```python
from build123d import *

# Parameters (mm, degrees)
BOSS_EXTRUDE1_DEPTH     = 35
CUT_EXTRUDE1_DEPTH      = 47.8508271
CUT_EXTRUDE1_DEPTH_BACK = 47.8508271
SKETCH2_R               = 12.8
SKETCH3_R               = 2
CUT_EXTRUDE2_DEPTH      = 7.5
SKETCH4_R               = 3.75
CUT_EXTRUDE3_DEPTH      = 16.5
SKETCH5_R               = 1.8
CUT_EXTRUDE4_DEPTH      = 22
SKETCH6_R               = 4
CUT_EXTRUDE5_DEPTH      = 2
SKETCH7_W               = 32
SKETCH7_H               = 6
CUT_EXTRUDE6_DEPTH      = 2
CUT_EXTRUDE7_DEPTH      = 47.850827224
CUT_EXTRUDE7_DEPTH_BACK = 47.850827224
SKETCH8_R               = 1.8
SKETCH9_R               = 3.75
CUT_EXTRUDE8_DEPTH      = 5
CUT_EXTRUDE9_DEPTH      = 8


with BuildPart() as part:
    # Sketch1 → Boss-Extrude1 (new, symmetric)
    with BuildSketch(Plane(origin=(0, 0, 0), x_dir=(0, 0, -1), z_dir=(1, 0, 0))):
        with BuildLine():
            Line((-19, 0.6), (19, 0.6))
            ThreePointArc((19, 0.6), (21.828427125, 1.771572875), (23, 4.6))
            Line((23, 4.6), (23, 17))
            ThreePointArc((23, 17), (21.828427125, 19.828427125), (19, 21))
            Line((19, 21), (-19, 21))
            ThreePointArc((-19, 21), (-21.828427125, 19.828427125), (-23, 17))
            Line((-23, 17), (-23, 4.6))
            ThreePointArc((-23, 4.6), (-21.828427125, 1.771572875), (-19, 0.6))
        make_face()
    extrude(amount=BOSS_EXTRUDE1_DEPTH, both=True)

    # Sketch2 → Cut-Extrude1 (cut, two sides: drawn at the far end of the back side and taken through both)
    with BuildSketch(Plane(origin=(0, 0, 0), x_dir=(0, 0, -1), z_dir=(1, 0, 0)).offset(-CUT_EXTRUDE1_DEPTH_BACK)):
        Circle(SKETCH2_R)
    extrude(amount=CUT_EXTRUDE1_DEPTH + CUT_EXTRUDE1_DEPTH_BACK, mode=Mode.SUBTRACT)

    # Sketch3 → Cut-Extrude2 (cut)
    with BuildSketch(Plane(origin=(0, 0.6, 0), x_dir=(1, 0, 0), z_dir=(0, 1, 0))):
        with Locations(Location((28, -17.5, 0), (0, 0, 228.590377891))):
            Circle(SKETCH3_R)
        with Locations(Location((28, 17.5, 0), (0, 0, 48.590377891))):
            Circle(SKETCH3_R)
        with Locations(Location((-28, -17.5, 0), (0, 0, 228.590377891))):
            Circle(SKETCH3_R)
        with Locations(Location((-28, 17.5, 0), (0, 0, 48.590377891))):
            Circle(SKETCH3_R)
    extrude(amount=CUT_EXTRUDE2_DEPTH, mode=Mode.SUBTRACT)

    # Sketch4 → Cut-Extrude3 (cut)
    with BuildSketch(Plane(origin=(0, 0, 0), x_dir=(1, 0, 0), z_dir=(0, 1, 0))):
        with Locations(Location((8.84, -8.84, 0), (0, 0, 90))):
            Circle(SKETCH4_R)
        with Locations(Location((8.84, 8.84, 0), (0, 0, 90))):
            Circle(SKETCH4_R)
        with Locations(Location((-8.84, -8.84, 0), (0, 0, 90))):
            Circle(SKETCH4_R)
        with Locations(Location((-8.84, 8.84, 0), (0, 0, 90))):
            Circle(SKETCH4_R)
    extrude(amount=CUT_EXTRUDE3_DEPTH, mode=Mode.SUBTRACT)

    # Sketch5 → Cut-Extrude4 (cut)
    with BuildSketch(Plane(origin=(0, 0, 0), x_dir=(1, 0, 0), z_dir=(0, 1, 0))):
        with Locations(Location((8.84, -8.84, 0), (0, 0, 90))):
            Circle(SKETCH5_R)
        with Locations(Location((8.84, 8.84, 0), (0, 0, 90))):
            Circle(SKETCH5_R)
        with Locations(Location((-8.84, -8.84, 0), (0, 0, 90))):
            Circle(SKETCH5_R)
        with Locations(Location((-8.84, 8.84, 0), (0, 0, 90))):
            Circle(SKETCH5_R)
    extrude(amount=CUT_EXTRUDE4_DEPTH, mode=Mode.SUBTRACT)

    # Sketch6 → Cut-Extrude5 (cut)
    with BuildSketch(Plane(origin=(0, 21, 0), x_dir=(1, 0, 0), z_dir=(0, 1, 0))):
        with Locations(Location((0, 0, 0), (0, 0, 270))):
            Circle(SKETCH6_R)
    extrude(amount=-CUT_EXTRUDE5_DEPTH, mode=Mode.SUBTRACT)

    # Sketch7 → Cut-Extrude6 (cut)
    with BuildSketch(Plane(origin=(0, 21, 0), x_dir=(1, 0, 0), z_dir=(0, 1, 0))):
        with Locations((19, 0)):
            Rectangle(SKETCH7_W, SKETCH7_H)
    extrude(amount=-CUT_EXTRUDE6_DEPTH, mode=Mode.SUBTRACT)

    # Sketch8 → Cut-Extrude7 (cut, two sides: drawn at the far end of the back side and taken through both)
    with BuildSketch(Plane.XY.offset(-CUT_EXTRUDE7_DEPTH_BACK)):
        with Locations((18, 0)):
            Circle(SKETCH8_R)
        with Locations((-18, 0)):
            Circle(SKETCH8_R)
    extrude(amount=CUT_EXTRUDE7_DEPTH + CUT_EXTRUDE7_DEPTH_BACK, mode=Mode.SUBTRACT)

    # Sketch9 → Cut-Extrude8 (cut)
    with BuildSketch(Plane.XY.offset(23)):
        with Locations((18, 0)):
            Circle(SKETCH9_R)
        with Locations((-18, 0)):
            Circle(SKETCH9_R)
    extrude(amount=-CUT_EXTRUDE8_DEPTH, mode=Mode.SUBTRACT)

    # Sketch10 → Cut-Extrude9 (cut)
    with BuildSketch(Plane.XY.offset(-23)):
        Polygon((20.85, 1.645448267), (18, 3.290896534), (15.15, 1.645448267), (15.15, -1.645448267), (18, -3.290896534), (20.85, -1.645448267), align=None)
        Polygon((-15.15, 1.645448267), (-18, 3.290896534), (-20.85, 1.645448267), (-20.85, -1.645448267), (-18, -3.290896534), (-15.15, -1.645448267), align=None)
    extrude(amount=CUT_EXTRUDE9_DEPTH, mode=Mode.SUBTRACT)


solid = part.part
```
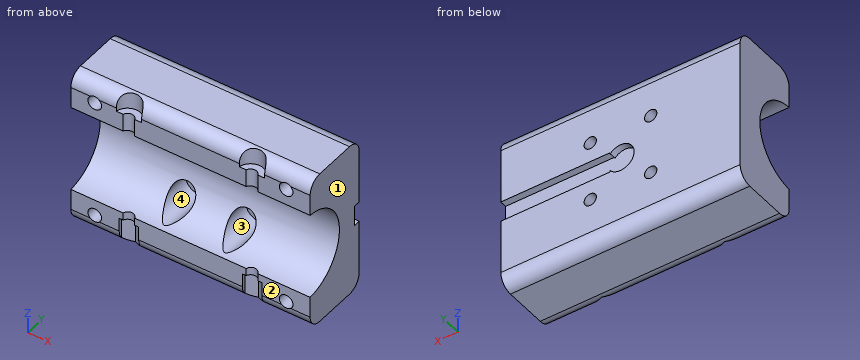
Geometry: final body of the model. Coordinates: model frame, mm. Face numbers are marked on the shaded views. Coordinates: 2 decimals unless noted, no trailing zeros. Write each loop counter-clockwise with the first axis right and the second up, starting at its lowest first coordinate (ties: lowest second). Pieces come first, ordered by that corner, then holes. Notation, with made-up numbers: M 38,58.5 L 94,58.5 A26 cw 94,80.5 Z; hole C -39.75,72 d11. An arc over 180 degrees is marked long. Use CSV: the item, a comma, the result in double quotes. Start each with the question number.
1. Cut plane A-A on y = 5.5. Return the cut outline in (x, z).
2. Cut plane B-B on z = -9. Return the cut outline in (x, y), plus the area to 3 significant figures.
3. Ray query, probe 1 along X at (y, z) = (19.9, 8.84); probe 2 along Z at (x, y) = (8.84, 8); probe 3 along X at (y, z) = (17.75, 7.5). Return the intervals inside material, ascending.
4. Cut plane C-C on y = 13.75. Return the cut outline in (x, z).
5. Cut plane D-D on x = -23. Return the cut outline in (y, z), plus the area to 3 significant figures.
6. Mould query, pull axis X, two halves, no side actions, for the marked faces 1, 2, 3 and 4. Classes: pulls with the +X half, pulls with the -X half, needs draft (parallel to the pull), parting line crosses it, or undercut.
7. First-contact query: P1, Ø3.5, axis at x = 18.5, y = 2, coming from the +Z side; P2, Ø4, axis at x = 12.5, z = 0, coming from the +Y side; P3, Ø3.5, axis at x = -28, z = 17.5, coming from the -Y side. Flat tips, straight axial feed; report the tip coordinate or a pass-through.
Entries:
1,outline,"M -35,-23 L 35,-23 L 35,-11.56 L 11.42,-11.56 A3.75 cw 6.26,-11.56 L -6.26,-11.56 A3.75 cw -11.42,-11.56 L -35,-11.56 Z; M -35,11.56 L -11.42,11.56 A3.75 cw -6.26,11.56 L 6.26,11.56 A3.75 cw 11.42,11.56 L 35,11.56 L 35,23 L -35,23 Z; hole C -28,-17.5 d4; hole C -28,17.5 d4; hole C 28,-17.5 d4; hole C 28,17.5 d4"
2,outline,"M -35,9.1 L -12.59,9.1 L -12.59,16.5 L -10.63,16.5 L -10.63,21 L -35,21 Z; M -7.05,16.5 L -5.09,16.5 L -5.09,9.1 L 5.09,9.1 L 5.09,16.5 L 7.05,16.5 L 7.05,21 L -7.05,21 Z; M 10.63,16.5 L 12.59,16.5 L 12.59,9.1 L 35,9.1 L 35,21 L 10.63,21 Z"
2,area,"690 mm²"
3,probe 1,"-35 to -10.64, -7.04 to 7.04, 10.64 to 35"
3,probe 2,"-23 to -12.59, 12.59 to 23"
3,probe 3,"-35 to -10.04, -7.64 to 7.64, 10.04 to 35"
4,outline,"M -35,-23 L 35,-23 L 35,23 L -35,23 Z; hole C -8.84,-8.84 d7.5; hole C -8.84,8.84 d7.5; hole C 8.84,-8.84 d7.5; hole C 8.84,8.84 d7.5"
5,outline,"M 0.6,-19 A4 ccw 4.6,-23 L 17,-23 A4 ccw 21,-19 L 21,19 A4 ccw 17,23 L 4.6,23 A4 ccw 0.6,19 L 0.6,12.79 A12.8 cw 0.6,-12.79 Z"
5,area,"683 mm²"
6,face 1,"pulls with the +X half"
6,face 2,"needs draft"
6,face 3,"undercut"
6,face 4,"undercut"
7,P1,"z = 22.91"
7,P2,"y = 19"
7,P3,"y = 8.1"
